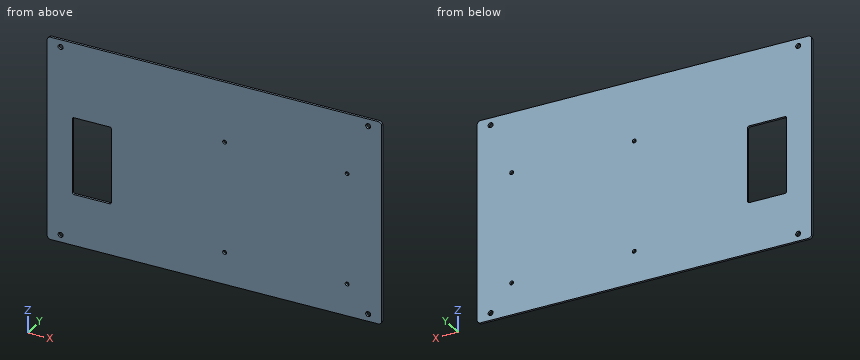
```python
from build123d import *

# Parameters (mm, degrees)
BASE_FLANGE2_DEPTH = 2
SKETCH2_R          = 2.25
CUT_EXTRUDE4_DEPTH = 10
CUT_EXTRUDE3_DEPTH = 10
CUT_EXTRUDE5_DEPTH = 10


# Sheet-metal steps are written as plain solids
with BuildPart() as part:
    # Sketch1 → Base-Flange2 (new body)
    with BuildSketch(Plane(origin=(0, 0, 0), x_dir=(1, 0, 0), z_dir=(0, 1, 0))):
        with BuildLine():
            Line((164.634355994, -145.755690278), (-129.365644006, -145.755690278))
            ThreePointArc((-129.365644006, -145.755690278), (-131.486964349, -144.877010621), (-132.365644006, -142.755690278))
            Line((-132.365644006, -142.755690278), (-132.365644006, 34.244309722))
            ThreePointArc((-132.365644006, 34.244309722), (-131.486964349, 36.365630066), (-129.365644006, 37.244309722))
            Line((-129.365644006, 37.244309722), (164.634355994, 37.244309722))
            ThreePointArc((164.634355994, 37.244309722), (166.755676338, 36.365630066), (167.634355994, 34.244309722))
            Line((167.634355994, 34.244309722), (167.634355994, -142.755690278))
            ThreePointArc((167.634355994, -142.755690278), (166.755676338, -144.877010621), (164.634355994, -145.755690278))
        make_face()
    extrude(amount=-BASE_FLANGE2_DEPTH)

    # Sketch2 → Cut-Extrude4 (cut)
    with BuildSketch(Plane(origin=(0, 0, 0), x_dir=(1, 0, 0), z_dir=(0, 1, 0))):
        with Locations(Location((-120.365644006, 30.744309722, 0), (0, 0, 270))):
            Circle(SKETCH2_R)
        with Locations(Location((-120.365644006, -139.255690278, 0), (0, 0, 270))):
            Circle(SKETCH2_R)
        with Locations(Location((155.634355994, -139.255690278, 0), (0, 0, 270))):
            Circle(SKETCH2_R)
        with Locations(Location((155.634355994, 30.744309722, 0), (0, 0, 270))):
            Circle(SKETCH2_R)
    extrude(amount=-CUT_EXTRUDE4_DEPTH, mode=Mode.SUBTRACT)

    # Sketch3 → Cut-Extrude3 (cut)
    with BuildSketch(Plane(origin=(0, 0, 0), x_dir=(1, 0, 0), z_dir=(0, 1, 0))):
        with BuildLine():
            Line((-107.836218664, -8.834875742), (-76.368346069, -8.834873742))
            ThreePointArc((-76.368346069, -8.834873742), (-75.307684442, -9.274214133), (-74.868344006, -10.334875742))
            Line((-74.868344006, -10.334875742), (-74.868344006, -76.822675742))
            ThreePointArc((-74.868344006, -76.822675742), (-75.307683834, -77.883335913), (-76.368344006, -78.322675742))
            Line((-76.368344006, -78.322675742), (-76.895069411, -78.322675742))
            Line((-76.895069411, -78.322675742), (-107.836218601, -78.322675742))
            Line((-107.836218601, -78.322675742), (-108.362944006, -78.322675742))
            ThreePointArc((-108.362944006, -78.322675742), (-109.423604177, -77.883335913), (-109.862944006, -76.822675742))
            Line((-109.862944006, -76.822675742), (-109.862944006, -10.334875742))
            ThreePointArc((-109.862944006, -10.334875742), (-109.423604177, -9.27421557), (-108.362944006, -8.834875742))
            Line((-108.362944006, -8.834875742), (-107.836218664, -8.834875742))
        make_face()
    extrude(amount=-CUT_EXTRUDE3_DEPTH, mode=Mode.SUBTRACT)

    # Sketch6 → Cut-Extrude5 (cut)
    with BuildSketch(Plane(origin=(0, 0, 0), x_dir=(1, 0, 0), z_dir=(0, 1, 0))):
        with BuildLine():
            add(Edge.make_bspline(
                [(28.521903533, -91.386017736), (28.521903533, -91.158613657), (28.431436566, -90.7038055), (28.044994377, -90.125453892), (27.466642769, -89.739011703), (26.784430533, -89.603311252), (26.102218297, -89.739011703), (25.52386669, -90.125453892), (25.1374245, -90.7038055), (25.00172405, -91.386017736), (25.1374245, -92.068229972), (25.52386669, -92.646581579), (26.102218297, -93.033023768), (26.784430533, -93.168724219), (27.466642769, -93.033023768), (28.044994377, -92.646581579), (28.431436566, -92.068229972), (28.521903533, -91.613421814), (28.521903533, -91.386017736)],
                knots=[0, 0, 0, 0, 0.0625, 0.125, 0.1875, 0.25, 0.3125, 0.375, 0.4375, 0.5, 0.5625, 0.625, 0.6875, 0.75, 0.8125, 0.875, 0.9375, 1, 1, 1, 1], degree=3))
        make_face()
        with BuildLine():
            add(Edge.make_bspline(
                [(138.471903533, 8.363982264), (138.471903533, 8.591386343), (138.381436566, 9.0461945), (137.994994377, 9.624546108), (137.416642769, 10.010988297), (136.734430533, 10.146688748), (136.052218297, 10.010988297), (135.47386669, 9.624546108), (135.0874245, 9.0461945), (134.95172405, 8.363982264), (135.0874245, 7.681770028), (135.47386669, 7.103418421), (136.052218297, 6.716976232), (136.734430533, 6.581275781), (137.416642769, 6.716976232), (137.994994377, 7.103418421), (138.381436566, 7.681770028), (138.471903533, 8.136578186), (138.471903533, 8.363982264)],
                knots=[0, 0, 0, 0, 0.0625, 0.125, 0.1875, 0.25, 0.3125, 0.375, 0.4375, 0.5, 0.5625, 0.625, 0.6875, 0.75, 0.8125, 0.875, 0.9375, 1, 1, 1, 1], degree=3))
        make_face()
        with BuildLine():
            add(Edge.make_bspline(
                [(28.521903533, 8.363982264), (28.521903533, 8.591386343), (28.431436566, 9.0461945), (28.044994377, 9.624546108), (27.466642769, 10.010988297), (26.784430533, 10.146688748), (26.102218297, 10.010988297), (25.52386669, 9.624546108), (25.1374245, 9.0461945), (25.00172405, 8.363982264), (25.1374245, 7.681770028), (25.52386669, 7.103418421), (26.102218297, 6.716976232), (26.784430533, 6.581275781), (27.466642769, 6.716976232), (28.044994377, 7.103418421), (28.431436566, 7.681770028), (28.521903533, 8.136578186), (28.521903533, 8.363982264)],
                knots=[0, 0, 0, 0, 0.0625, 0.125, 0.1875, 0.25, 0.3125, 0.375, 0.4375, 0.5, 0.5625, 0.625, 0.6875, 0.75, 0.8125, 0.875, 0.9375, 1, 1, 1, 1], degree=3))
        make_face()
        with BuildLine():
            add(Edge.make_bspline(
                [(138.471903533, -91.386017736), (138.471903533, -91.158613657), (138.381436566, -90.7038055), (137.994994377, -90.125453892), (137.416642769, -89.739011703), (136.734430533, -89.603311252), (136.052218297, -89.739011703), (135.47386669, -90.125453892), (135.0874245, -90.7038055), (134.95172405, -91.386017736), (135.0874245, -92.068229972), (135.47386669, -92.646581579), (136.052218297, -93.033023768), (136.734430533, -93.168724219), (137.416642769, -93.033023768), (137.994994377, -92.646581579), (138.381436566, -92.068229972), (138.471903533, -91.613421814), (138.471903533, -91.386017736)],
                knots=[0, 0, 0, 0, 0.0625, 0.125, 0.1875, 0.25, 0.3125, 0.375, 0.4375, 0.5, 0.5625, 0.625, 0.6875, 0.75, 0.8125, 0.875, 0.9375, 1, 1, 1, 1], degree=3))
        make_face()
    extrude(amount=-CUT_EXTRUDE5_DEPTH, mode=Mode.SUBTRACT)


solid = part.part
```
Work out the finished part from the listing and answer in its coordinate system (mm). Give positions to 0.01 mm unless a question says otherwise; leave off trailing zeros. Write each loop counter-clockwise with the first axis right and the second up, starting at its lowest first coordinate (ties: lowest second). Pieces come first, ordered by that corner, then holes.
(1) The part is cut by section A-A on x = -90. Write down the section's boundary in (y, z), plus the area to 3 significant figures.
Final values:
outline: (-2, -37.24) - (0, -37.24) - (0, 8.83) - (-2, 8.83) - close; (-2, 78.32) - (0, 78.32) - (0, 145.76) - (-2, 145.76) - close
area: 227 mm2
(2) The part is cut by section B-B on z = 50. Write down the section's boundary in (x, y).
Final values:
outline: (-132.37, -2) - (-109.86, -2) - (-109.86, 0) - (-132.37, 0) - close; (-74.87, -2) - (167.63, -2) - (167.63, 0) - (-74.87, 0) - close
(3) Straight lines are drawn through the part: line 1 (Z direction, x = -91, y = -0.5); line 2 (X direction, y = -1.8, z = 62.5). For each, find the intervals that lie inside material, in ascending order.
Final values:
line 1: z = -37.24 to 8.83, 78.32 to 145.76
line 2: x = -132.37 to -109.86, -74.87 to 167.63
(4) The part is cut by section C-C on y = -0.85. Count the separate pieces of the cut face and the enclosed holes in it, plus the area to 3 significant figures.
Final values:
separate pieces: 1
enclosed holes: 9
area: 52,400 mm2
(5) Flat-ended cylindrical pins translate along their axes: pin 1 Ø6 at (x, z) = (155.63, -30.74) entering from +Y; pin 2 Ø3.5 at (x, z) = (-120.37, 139.26) entering from +Y. Find the tip coordinate at first contact, or state that the pin passes through.
Final values:
pin 1: stops at y = 0
pin 2: passes through
